Could you check a few things on this drawing? It's one solid part, dimensions in mm from its lowest x, y, z. A direction names the side the tool comes from. Round coordinates to 2 decimals unless told otherwise and drop trailing zeros. Order: outer loops, then holes, each group sorted by start corner. A loop starts at its lowest first (then second) coordinate and runs counter-clockwise, first axis right, second up.
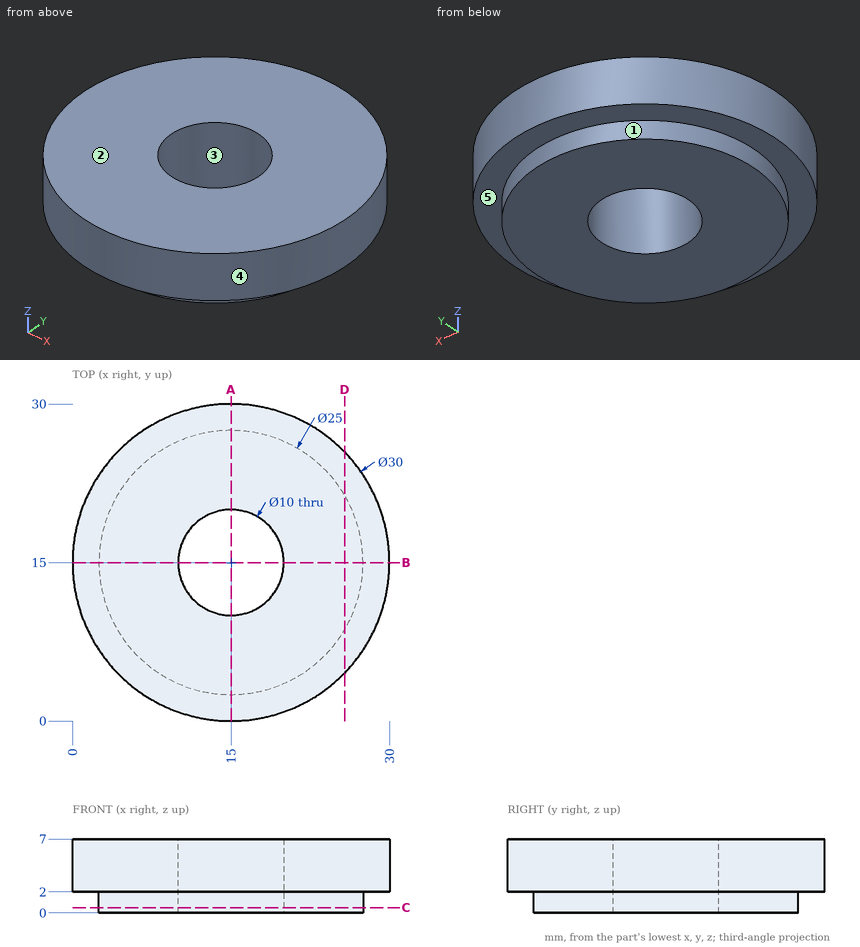
1) If we section it at A-A (x = 15): Write out the boundary of the cut face in (y, z).
2) If we section it at C-C (z = 0.5): Write out the boundary of the cut face in (x, y).
3) We'd pull the mould along Y, two halves only. Please class the marked faces 3, 4 and 5: +Y half, -Y half, draft (parallel to the pull), parting line (faces both ways), or undercut.
4) If we section it at D-D (x = 25.75): Write out the boundary of the cut face in (y, z), plus the area to 3 significant figures.
5) I need wall thicknesses on line 1 (Y direction, x = 15, z = 4.5); line 2 (Z direction, x = 5.75, y = 26.75); line 3 (Y direction, x = 8, z = 2.5). Which ranges of each line are inside material? Lowest first, please.
6) For the marked faces 1 and 2, which set-ups out of +Z, -Z, +X, -X, +Y, -Y let a thin tool reach every point of the face, with its end or its side?
7) I'm going to push flat-ended pins straight in: pin 1 (2 mm diameter, centred on y = 22, z = 5, fed in from -X); pin 2 (2 mm diameter, centred on y = 24, z = 1.5, fed in from -X); pin 3 (2 mm diameter, centred on y = 10.5, z = 5, fed in from +X). Where does each tip first touch, or does it pass through?
Solutions:
1. outline: (0, 2) - (2.5, 2) - (2.5, 0) - (10, 0) - (10, 7) - (0, 7) - close; (20, 0) - (27.5, 0) - (27.5, 2) - (30, 2) - (30, 7) - (20, 7) - close
2. outline: circle Ø25 at (15, 15); hole circle Ø10 at (15, 15)
3. face 3: undercut
3. face 4: parting line
3. face 5: draft
4. outline: (4.54, 2) - (8.62, 2) - (8.62, 0) - (21.38, 0) - (21.38, 2) - (25.46, 2) - (25.46, 7) - (4.54, 7) - close
4. area: 130 mm2
5. line 1: y = 0 to 10, 20 to 30
5. line 2: z = 2 to 7
5. line 3: y = 1.73 to 28.27
6. face 1: -Z
6. face 2: +Z, +X, -X, +Y, -Y
7. pin 1: stops at x = 1.25
7. pin 2: stops at x = 2.4
7. pin 3: stops at x = 29.59
